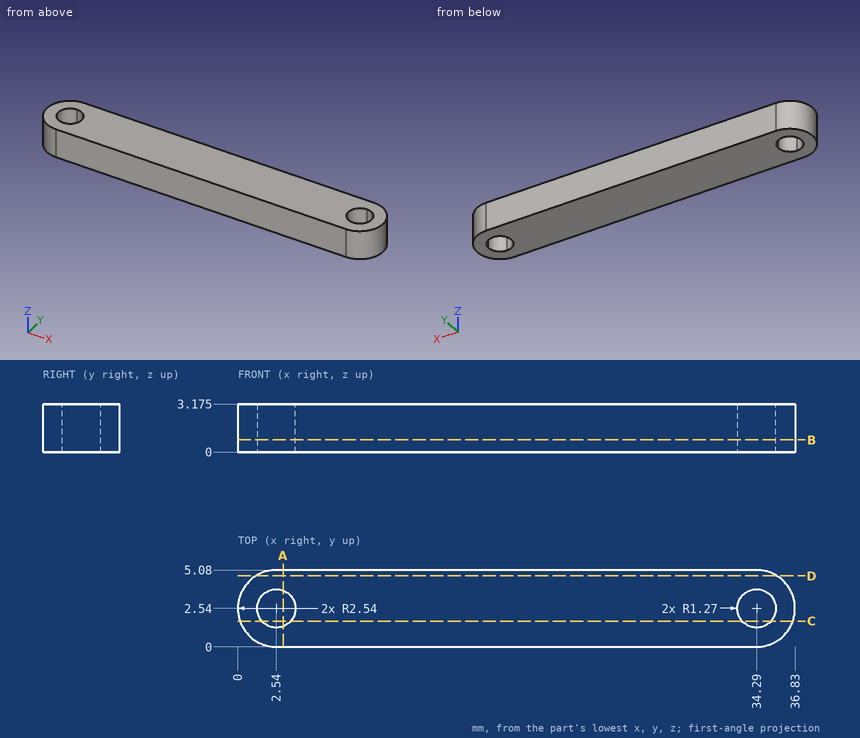
For this review, use the dimensioned drawing (mm, ordinates from the lowest corner) and the shaded views. Coordinates: 2 decimals unless noted, no trailing zeros. Write each loop counter-clockwise with the first axis right and the second up, starting at its lowest first coordinate (ties: lowest second). Pieces come first, ordered by that corner, then holes. Notation, with made-up numbers: (9, 36) -> (39, 36) arc R5 cw to (39, 45) -> close; hole circle Ø5 at (68, 18). An arc over 180 degrees is marked (long way). Put each result on its own line as item: value.
Q1. Take a section at A-A, the plane x = 3. State the section outline as (y, z) points (3 decimals), then the cut area to 3 significant figures.
From the geometry:
outline: (0, 0) -> (1.356, 0) -> (1.356, 3.175) -> (0, 3.175) -> close; (3.724, 0) -> (5.08, 0) -> (5.08, 3.175) -> (3.724, 3.175) -> close
area: 8.61 mm2
Q2. Wall thickness on L1, parallel to X at y = 1.8, z = 2.5; L2, parallel to X at y = 3.2, z = 0.6; L3, parallel to Y at x = 3, z = 0.9: over which ranges is each line inside the solid? List them lowest first.
From the geometry:
L1: x = 0.11 to 1.51, 3.57 to 33.26, 35.32 to 36.72
L2: x = 0.09 to 1.45, 3.63 to 33.2, 35.38 to 36.74
L3: y = 0 to 1.36, 3.72 to 5.08
Q3. Take a section at C-C, the plane y = 1.7. State the section outline as (x, z) points (3 decimals).
From the geometry:
outline: (0.143, 0) -> (1.587, 0) -> (1.587, 3.175) -> (0.143, 3.175) -> close; (3.493, 0) -> (33.337, 0) -> (33.337, 3.175) -> (3.493, 3.175) -> close; (35.243, 0) -> (36.687, 0) -> (36.687, 3.175) -> (35.243, 3.175) -> close
Q4. Take a section at B-B, the plane z = 0.8. State the section outline as (x, y) points, then the cut area to 3 significant figures.
From the geometry:
outline: (2.54, 0) -> (34.29, 0) arc R2.54 ccw to (34.29, 5.08) -> (2.54, 5.08) arc R2.54 ccw to start; hole (2.54, 1.27) arc R1.27 ccw to (3.81, 2.54) arc R1.27 ccw to (2.54, 3.81) arc R1.27 ccw to start; hole (34.29, 1.27) arc R1.27 ccw to (35.56, 2.54) arc R1.27 ccw to (34.29, 3.81) arc R1.27 ccw to start
area: 171 mm2
Q5. Take a section at D-D, the plane y = 4.7. State the section outline as (x, z) points (3 decimals), then the cut area to 3 significant figures.
From the geometry:
outline: (1.204, 0) -> (35.626, 0) -> (35.626, 3.175) -> (1.204, 3.175) -> close
area: 109 mm2
